Print and shaded views of the part. All mm, measured from the part's lowest x, y and z. Give positions to 0.01 mm unless a question says otherwise; leave off trailing zeros. Use one line per item in the form item = value. Start each with the question number.
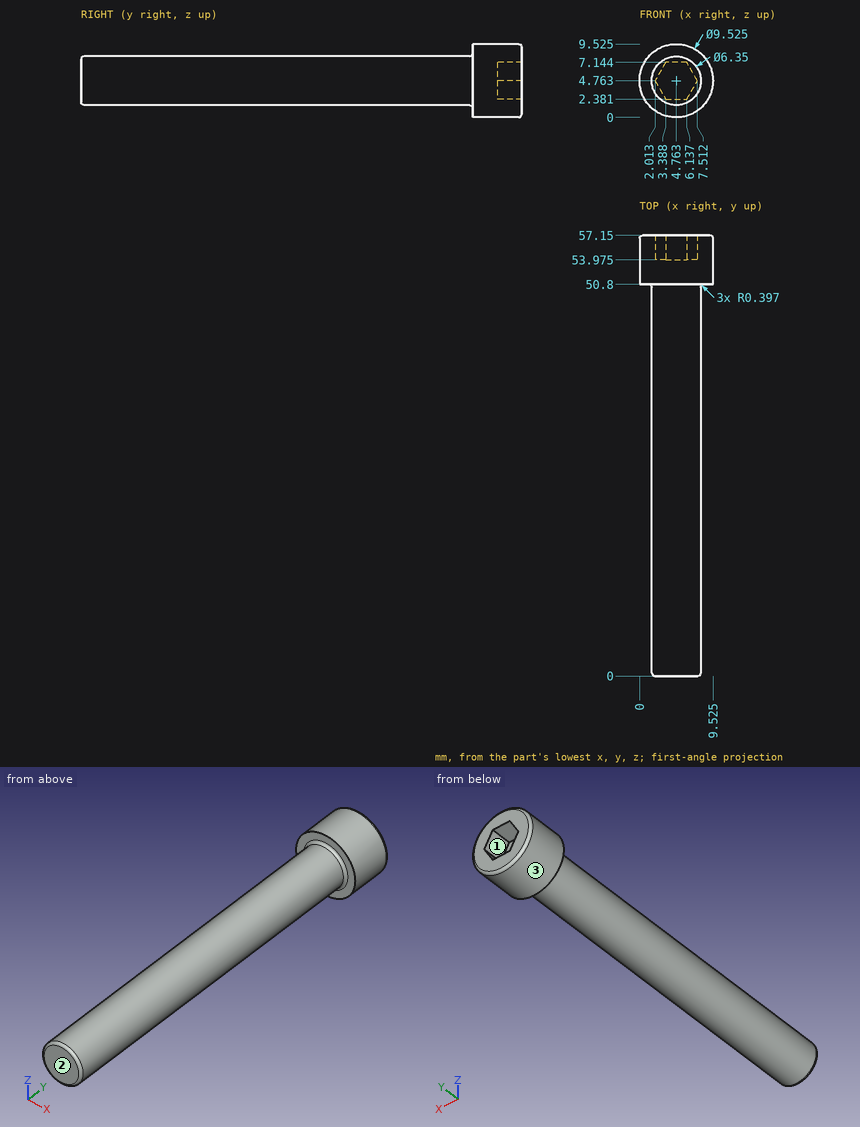
(1) Pin check, flat tips, straight feed: pin 1 Ø1.5 at (y, z) = (40, 1.5) entering from +X (1 decimal); pin 2 Ø3 at (y, z) = (42.5, 4.5) entering from -X; pin 3 Ø0.8 at (x, y) = (5.5, 55.5) entering from +Z. Stop position of each tip, or through.
(2) Two-plate mould, pull along Z, no slides. Class the marked faces 1, 2 and 3: +Z half, -Z half, draft (parallel to the pull), parting line (faces both ways), or undercut.
(3) Wall check: line 1 (Y direction, x = 5.75, z = 5.5) (1 decimal); line 2 (Y direction, x = 5.5, z = 8.25); line 3 (X direction, y = 24, z = 4.75). Give the ranges that are in metal, low to high. Write a range as from..to.
Solution:
q1.pin_1 = 6.7
q1.pin_2 = 1.59
q1.pin_3 = 9.51
q2.face_1 = undercut
q2.face_2 = draft
q2.face_3 = parting line
q3.line_1 = 0..54
q3.line_2 = 50.8..57.15
q3.line_3 = 1.59..7.94
